Could you check a few things on this drawing? It's one solid part, dimensions in mm from its lowest x, y, z. Give positions to 0.01 mm unless a question says otherwise; leave off trailing zeros. Loops run counter-clockwise (first coordinate to the right, second up) from the corner with the lowest first, then second, coordinate; pieces in that order, holes last.
1. I need wall thicknesses on line 1 along X through (y, z) = (61, 8) (3 decimals); line 2 along X through (y, z) = (59, 8.75); line 3 along Y through (x, z) = (8, 8.5) (3 decimals). Which ranges of each line are inside material? Lowest first, please.
2. Imagine slicing it at D-D (x = 19). List the corners of the cut face in (y, z) for me, plus the area to 3 significant figures.
3. Imagine slicing it at B-B (x = 32). List the corners of the cut face in (y, z) for me (3 decimals), plus the area to 3 significant figures.
4. Thinking about a two-plate mould opening in Y: for the marked faces 1, 2 and 3, which applies, +Y half, -Y half, draft (parallel to the pull), parting line (faces both ways), or undercut?
5. For P1, Ø12, axis at x = 25.5, y = 13, coming from the -Z side; P2, Ø4.5, axis at x = 8, y = 61, coming from the -Z side; P3, Ø6, axis at x = 8, y = 21, coming from the -Z side, each with a flat end and sliding along its axis, tell me the tip position at first contact or that it passes through.
6. Imagine slicing it at A-A (y = 75). List the corners of the cut face in (x, z) for me (3 decimals).
7. Imagine slicing it at C-C (z = 7.5). Count the separate pieces of the cut face and the enclosed holes in it, plus the area to 3 significant figures.
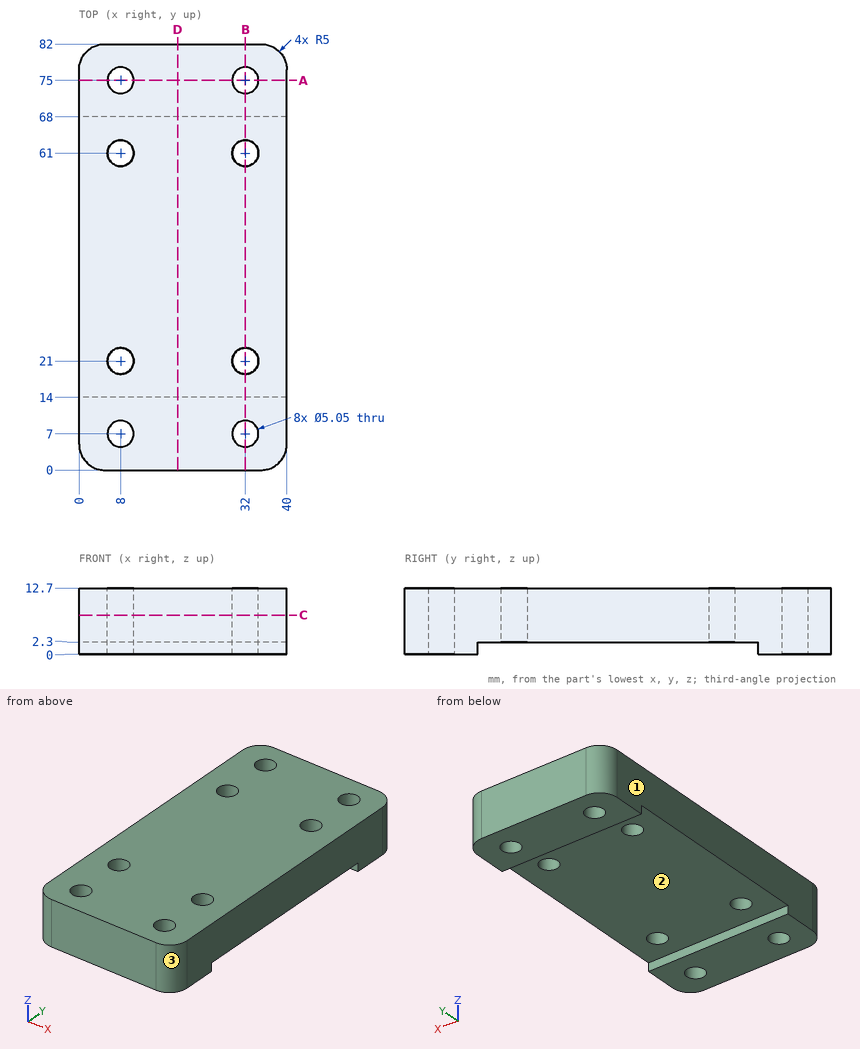
Derived:
1. line 1: x = 0 to 5.475, 10.525 to 29.475, 34.525 to 40
1. line 2: x = 0 to 6.46, 9.54 to 30.46, 33.54 to 40
1. line 3: y = 0 to 4.475, 9.525 to 18.475, 23.525 to 58.475, 63.525 to 72.475, 77.525 to 82
2. outline: (0, 0) - (14, 0) - (14, 2.3) - (68, 2.3) - (68, 0) - (82, 0) - (82, 12.7) - (0, 12.7) - close
2. area: 917 mm2
3. outline: (0, 0) - (4.475, 0) - (4.475, 12.7) - (0, 12.7) - close; (9.525, 0) - (14, 0) - (14, 2.3) - (18.475, 2.3) - (18.475, 12.7) - (9.525, 12.7) - close; (23.525, 2.3) - (58.475, 2.3) - (58.475, 12.7) - (23.525, 12.7) - close; (63.525, 2.3) - (68, 2.3) - (68, 0) - (72.475, 0) - (72.475, 12.7) - (63.525, 12.7) - close; (77.525, 0) - (82, 0) - (82, 12.7) - (77.525, 12.7) - close
3. area: 684 mm2
4. face 1: draft
4. face 2: undercut
4. face 3: -Y half
5. P1: stops at z = 0
5. P2: passes through
5. P3: stops at z = 2.3
6. outline: (0, 0) - (5.475, 0) - (5.475, 12.7) - (0, 12.7) - close; (10.525, 0) - (29.475, 0) - (29.475, 12.7) - (10.525, 12.7) - close; (34.525, 0) - (40, 0) - (40, 12.7) - (34.525, 12.7) - close
7. separate pieces: 1
7. enclosed holes: 8
7. area: 3,100 mm2
